Part print with two shaded views. Sizes in mm from the minimum x, y, z corner. Round coordinates to 2 decimals unless told otherwise and drop trailing zeros. Write each loop counter-clockwise with the first axis right and the second up, starting at its lowest first coordinate (ties: lowest second). Pieces come first, ordered by that corner, then holes. Notation, with made-up numbers: (-33, 64.5) -> (-1, 64.5) arc R26 ccw to (-1, 100.5) -> close; hole circle Ø11 at (65.5, 46). An arc over 180 degrees is marked (long way). Answer in a Markdown table with one row per item. Add a question column.
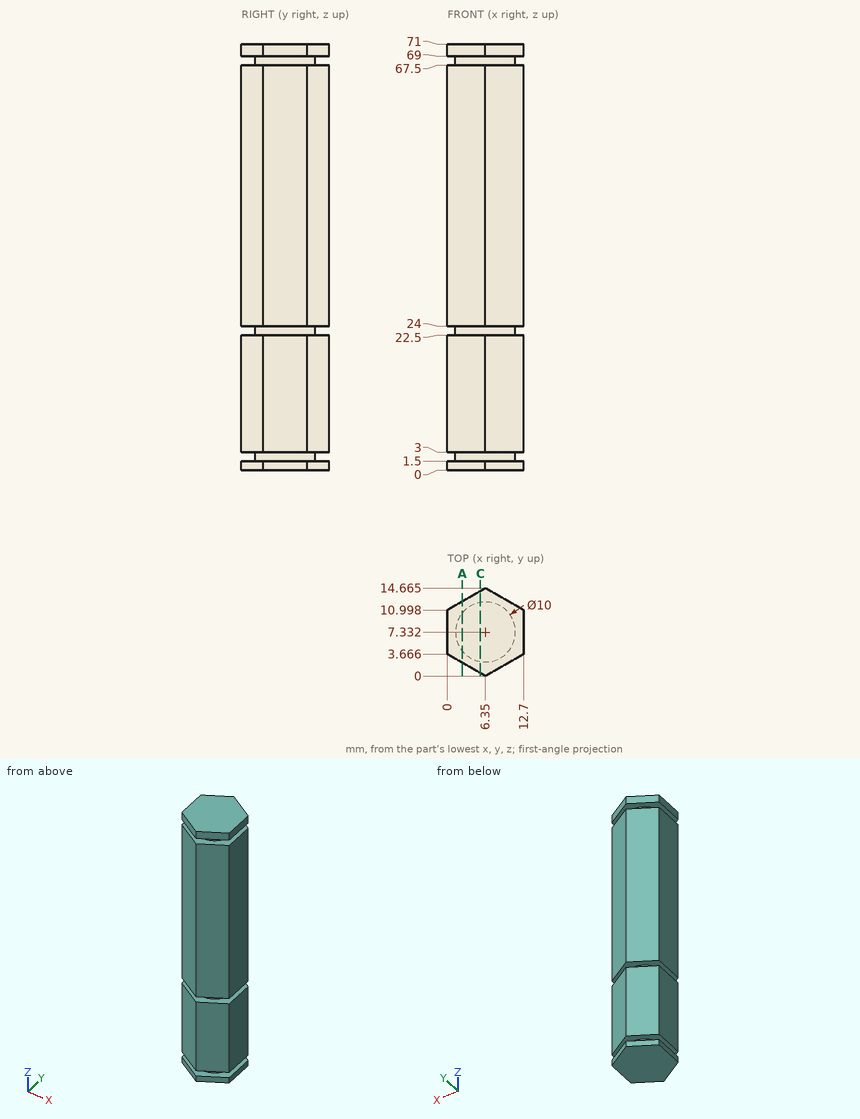
Item 1: Pin check, flat tip, straight feed: pin 1 (6 mm diameter, centred on x = 3.5, z = 46.5, fed in from -Y). Stop position of the tip, or through.
Item 2: Drill centre lines: probe 1 along Z at (x, y) = (1.5, 10.25); probe 2 along Y at (x, z) = (1.25, 44) (1 decimal); probe 3 along Y at (x, z) = (5.5, 33.5) (1 decimal). Where is each one in solid material? Low to high.
Item 3: Saw through at A-A on x = 2.5. Give the cut face in (y, z), then the cut area to 3 significant figures.
Item 4: Saw through at C-C on x = 5.5. Give the cut face in (y, z) (1 decimal).
Recorded:
| question | item | result |
|---|---|---|
| 1 | pin 1 | y = 0 |
| 2 | probe 1 | 0 to 1.5, 3 to 22.5, 24 to 67.5, 69 to 71 |
| 2 | probe 2 | 2.9 to 11.7 |
| 2 | probe 3 | 0.5 to 14.2 |
| 3 | outline | (2.22, 0) -> (12.44, 0) -> (12.44, 1.5) -> (10.52, 1.5) -> (10.52, 3) -> (12.44, 3) -> (12.44, 22.5) -> (10.52, 22.5) -> (10.52, 24) -> (12.44, 24) -> (12.44, 67.5) -> (10.52, 67.5) -> (10.52, 69) -> (12.44, 69) -> (12.44, 71) -> (2.22, 71) -> (2.22, 69) -> (4.14, 69) -> (4.14, 67.5) -> (2.22, 67.5) -> (2.22, 24) -> (4.14, 24) -> (4.14, 22.5) -> (2.22, 22.5) -> (2.22, 3) -> (4.14, 3) -> (4.14, 1.5) -> (2.22, 1.5) -> close |
| 3 | area | 708 mm2 |
| 4 | outline | (0.5, 0) -> (14.2, 0) -> (14.2, 1.5) -> (12.3, 1.5) -> (12.3, 3) -> (14.2, 3) -> (14.2, 22.5) -> (12.3, 22.5) -> (12.3, 24) -> (14.2, 24) -> (14.2, 67.5) -> (12.3, 67.5) -> (12.3, 69) -> (14.2, 69) -> (14.2, 71) -> (0.5, 71) -> (0.5, 69) -> (2.4, 69) -> (2.4, 67.5) -> (0.5, 67.5) -> (0.5, 24) -> (2.4, 24) -> (2.4, 22.5) -> (0.5, 22.5) -> (0.5, 3) -> (2.4, 3) -> (2.4, 1.5) -> (0.5, 1.5) -> close |
